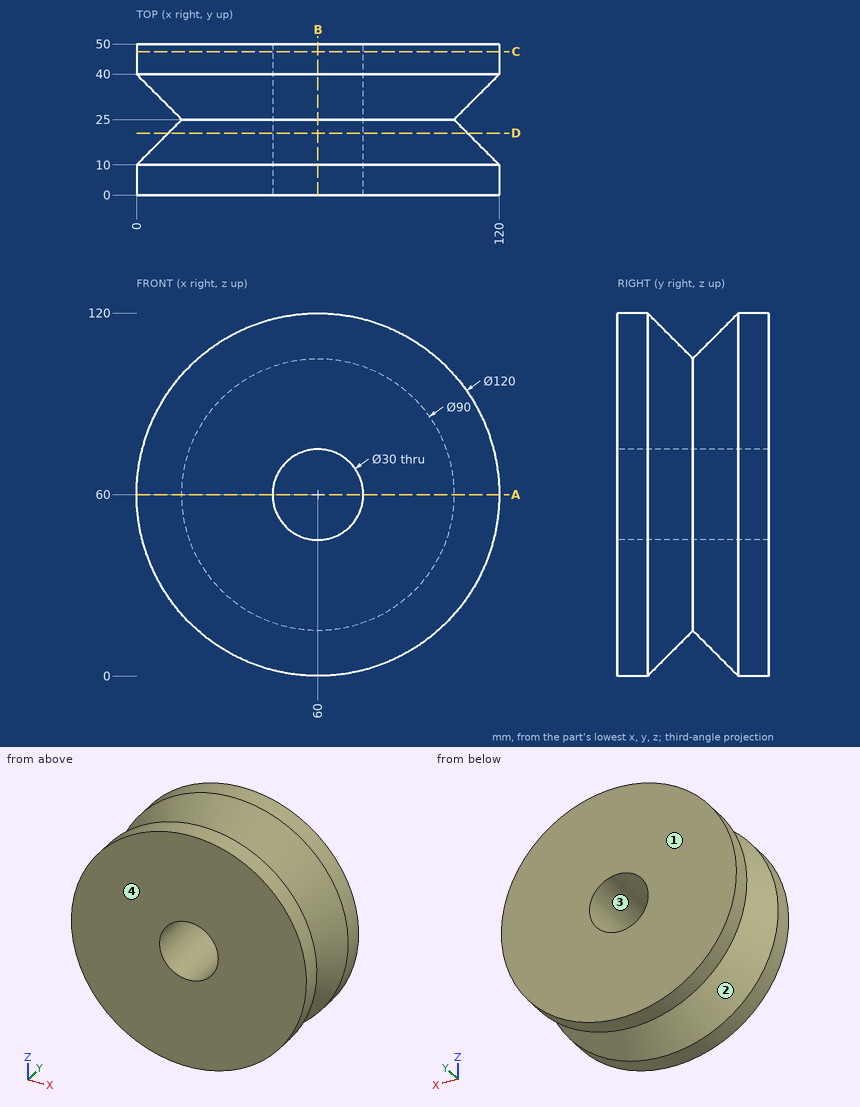
For this review, use the dimensioned drawing (mm, ordinates from the lowest corner) and the shaded views. Coordinates: 2 decimals unless noted, no trailing zeros. Loops run counter-clockwise (first coordinate to the right, second up) from the corner with the lowest first, then second, coordinate; pieces in that order, holes last. Notation, with made-up numbers: (17.25, 89.25) -> (63.25, 89.25) arc R35 cw to (63.25, 123.25) -> close; hole circle Ø3 at (64, 22). An arc over 180 degrees is marked (long way). Use a Markdown table: item, result. Add a question column.
Item 1: The part is to be moulded in two halves that separate along Y. For the marked faces 1, 2, 3 and 4, say which applies: +Y half, -Y half, draft (parallel to the pull), parting line (faces both ways), or undercut.
Item 2: We need section B-B, the plane x = 60. Write out the cut boundary in (y, z).
Item 3: Clearance check with flat-ended pins moving along their axes: P1, Ø8, axis at y = 22, z = 23, coming from the +X side; P2, Ø8, axis at x = 23.5, y = 6, coming from the -Z side; P3, Ø1.5, axis at x = 85.5, y = 6.5, coming from the +Z side. State where each tip first meets the part, or that it passes through.
Item 4: We need section D-D, the plane y = 20.5. Write out the cut boundary in (x, z), and give its area (3 significant figures).
Item 5: We need section A-A, the plane z = 60. Write out the cut boundary in (x, y).
Item 6: Wall thickness on L1, parallel to Z at x = 60, y = 15.5; L2, parallel to X at y = 9, z = 52; L3, parallel to Z at x = 60, y = 23: over which ranges is each line inside the solid? List them lowest first. Write a range as from..to.
Item 7: We need section C-C, the plane y = 47.5. Write out the cut boundary in (x, z), and give its area (3 significant figures).
Numbers:
| question | item | result |
|---|---|---|
| 1 | face 1 | +Y half |
| 1 | face 2 | undercut |
| 1 | face 3 | draft |
| 1 | face 4 | -Y half |
| 2 | outline | (0, 0) -> (10, 0) -> (25, 15) -> (40, 0) -> (50, 0) -> (50, 45) -> (0, 45) -> close; (0, 75) -> (50, 75) -> (50, 120) -> (40, 120) -> (25, 105) -> (10, 120) -> (0, 120) -> close |
| 3 | P1 | stops at x = 97.75 |
| 3 | P2 | stops at z = 9.56 |
| 3 | P3 | stops at z = 114.66 |
| 4 | outline | circle Ø99 at (60, 60); hole circle Ø30 at (60, 60) |
| 4 | area | 6,990 mm^2 |
| 5 | outline | (0, 0) -> (45, 0) -> (45, 50) -> (0, 50) -> (0, 40) -> (15, 25) -> (0, 10) -> close; (75, 0) -> (120, 0) -> (120, 10) -> (105, 25) -> (120, 40) -> (120, 50) -> (75, 50) -> close |
| 6 | L1 | z = 5.5..45, 75..114.5 |
| 6 | L2 | x = 0.54..47.31, 72.69..119.46 |
| 6 | L3 | z = 13..45, 75..107 |
| 7 | outline | circle Ø120 at (60, 60); hole circle Ø30 at (60, 60) |
| 7 | area | 10,600 mm^2 |
